Here's how the part is built. I have some questions about the finished solid (model axes, mm). Face numbers are marked on the shaded views. A direction names the side the tool comes from. Round coordinates to 2 decimals unless told otherwise and drop trailing zeros. Write each loop counter-clockwise with the first axis right and the second up, starting at its lowest first coordinate (ties: lowest second). Pieces come first, ordered by that corner, then holes. Notation, with made-up numbers: (63, 45) - (122, 45) arc R30 ccw to (122, 70) - close; hole circle Ø9 at (37, 16). An arc over 180 degrees is marked (long way). One line per item, written item: value. Start each with the question number.
Item 1: For the marked faces 4 and 5, which set-ups out of +Z, -Z, +X, -X, +Y, -Y let a thin tool reach every point of the face, with its end or its side?
Item 2: For P1, Ø12, axis at x = 30.5, y = 45.5, coming from the -Z side, with a flat end and sliding along its axis, tell me the tip position at first contact or that it passes through.
Item 3: Imagine slicing it at A-A, the plane x = 168. Please give me the cut outline in (y, z).
Item 4: Imagine slicing it at D-D, the plane y = 59. Please give me the cut outline in (x, z), then the cut area to 3 significant figures.
Item 5: Imagine slicing it at C-C, the plane z = 9. Please give me the cut outline in (x, y).
Item 6: If I drill on line 1 (X direction, y = 75, z = 8); line 2 (Y direction, x = 111.5, z = 14.75); line 3 (Y direction, x = 8, z = 4), over which ranges is the centre line in solid material (lowest first)?
Item 7: Thinking about a two-plate mould opening in Y: for the marked faces 1, 2 and 3, which applies, released by +Y, released by -Y, zero draft, split by the parting line, or undercut?
Item 8: Imagine slicing it at B-B, the plane y = 75. Please give me the cut outline in (x, z), then the cut area to 4 significant figures.
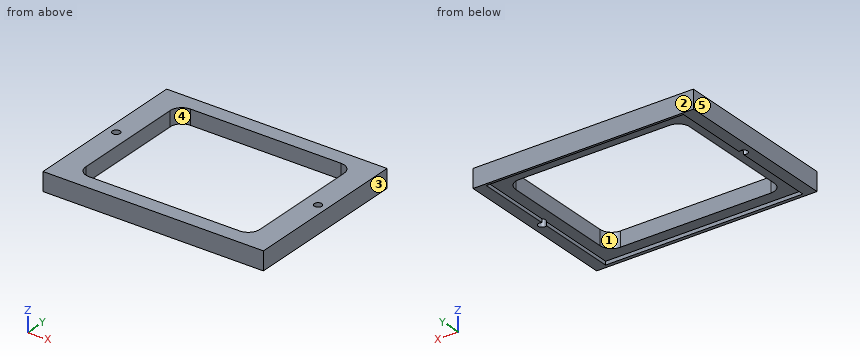
```python
from build123d import *

# Parameters (mm, degrees)
CYLINDER_R     = 3.25
CYLINDER_DEPTH = 26
ARRAY_X_COUNT  = 2
ARRAY_X_PITCH  = 174
BOX002_W       = 170
BOX002_H       = 140
BOX002_DEPTH   = 3
BOX001_W       = 150
BOX001_H       = 119
BOX001_DEPTH   = 16
BOX_W          = 190
BOX_H          = 145
BOX_DEPTH      = 16
FILLET_R       = 10


with BuildPart() as array:
    # Cylinder → Cylinder (new body)
    with BuildSketch(Plane(origin=(8, 75, 0), x_dir=(1, 0, 0), z_dir=(0, 0, 1))):
        Circle(CYLINDER_R)
    extrude(amount=CYLINDER_DEPTH)

    # Array X: Array ×2


with BuildPart() as array_1:
    add(array.part)
    with Locations(*[(i * ARRAY_X_PITCH, 0, 0) for i in range(1, ARRAY_X_COUNT)]):
        add(array.part)


with BuildPart() as cubo001:
    # Box002 → Box002 (new body)
    with BuildSketch(Plane(origin=(10, 3, 0), x_dir=(1, 0, 0), z_dir=(0, 0, 1))):
        with Locations((85, 70)):
            Rectangle(BOX002_W, BOX002_H)
    extrude(amount=BOX002_DEPTH)


with BuildPart() as fusion:
    # Box001 → Box001 (new body)
    with BuildSketch(Plane(origin=(20, 13, 0), x_dir=(1, 0, 0), z_dir=(0, 0, 1))):
        with Locations((75, 59.5)):
            Rectangle(BOX001_W, BOX001_H)
    extrude(amount=BOX001_DEPTH)

    # Fusion: union Cubo001
    add(cubo001.part)


with BuildPart() as fillet_body:
    # Box → Box (new body)
    with BuildSketch(Plane.XY):
        with Locations((95, 72.5)):
            Rectangle(BOX_W, BOX_H)
    extrude(amount=BOX_DEPTH)

    # Cut: cut Fusion
    add(fusion.part, mode=Mode.SUBTRACT)

    # Cut001: cut Array
    add(array_1.part, mode=Mode.SUBTRACT)

    # Fillet
    fillet_edges = [fillet_body.edges().sort_by_distance(p)[0] for p in [
        (170, 132, 9.5),
        (20, 132, 9.5),
        (170, 13, 9.5),
        (20, 13, 9.5),
    ]]
    fillet(fillet_edges, radius=FILLET_R)


solid = fillet_body.part
```
Values follow:
1. face 4: +Z, -Z
1. face 5: +Z, -Z, -X, +Y, -Y
2. P1: passes through
3. outline: (0, 0) - (3, 0) - (3, 3) - (17, 3) - (17, 16) - (0, 16) - close; (128, 3) - (143, 3) - (143, 0) - (145, 0) - (145, 16) - (128, 16) - close
4. outline: (0, 0) - (10, 0) - (10, 3) - (20, 3) - (20, 16) - (0, 16) - close; (170, 3) - (180, 3) - (180, 0) - (190, 0) - (190, 16) - (170, 16) - close
4. area: 580 mm^2
5. outline: (0, 0) - (190, 0) - (190, 145) - (0, 145) - close; hole circle Ø6.5 at (8, 75); hole (20, 23) arc R10 ccw to (30, 13) - (160, 13) arc R10 ccw to (170, 23) - (170, 122) arc R10 ccw to (160, 132) - (30, 132) arc R10 ccw to (20, 122) - close; hole circle Ø6.5 at (182, 75)
6. line 1: x = 0 to 4.75, 11.25 to 20, 170 to 178.75, 185.25 to 190
6. line 2: y = 0 to 13, 132 to 145
6. line 3: y = 0 to 71.75, 78.25 to 145
7. face 1: undercut
7. face 2: released by +Y
7. face 3: zero draft
8. outline: (0, 0) - (4.75, 0) - (4.75, 16) - (0, 16) - close; (11.25, 3) - (20, 3) - (20, 16) - (11.25, 16) - close; (170, 3) - (178.75, 3) - (178.75, 16) - (170, 16) - close; (185.25, 0) - (190, 0) - (190, 16) - (185.25, 16) - close
8. area: 379.5 mm^2
